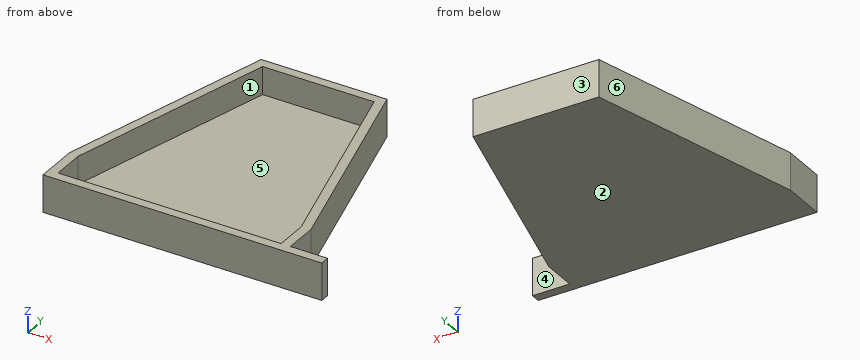
from build123d import *

# Parameters (mm, degrees)
F2_DEPTH = 3.175
F3_DEPTH = 12.7
F4_W     = 3.175
F4_H     = 12.7
F5_DEPTH = 12.7


with BuildPart() as f2:
    # F0 (on Top) → F2 (new body)
    with BuildSketch(Plane.XY):
        Polygon((-38.1, -30.1625), (-38.1, -41.275), (38.1, -41.275), (38.1, -30.1625), (19.05, 41.275), (-19.05, 41.275), align=None)
    extrude(amount=F2_DEPTH)

    # F1 (on face) → F3 (join)
    with BuildSketch(Plane.XY):
        Polygon((21.489284, 44.45), (-21.489284, 44.45), (-41.275, -29.746436), (-41.275, -44.45), (41.275, -44.45), (41.275, -29.746436), align=None)
        Polygon((-38.1, -41.275), (-38.1, -30.1625), (-19.05, 41.275), (19.05, 41.275), (38.1, -30.1625), (38.1, -41.275), align=None, mode=Mode.SUBTRACT)
    extrude(amount=F3_DEPTH)

    # F4 (on face) → F5 (join)
    with BuildSketch(Plane.YZ.offset(41.275)):
        with Locations((-42.8625, 6.35)):
            Rectangle(F4_W, F4_H)
    extrude(amount=F5_DEPTH)


solid = f2.part
Read the model definition and answer for the solid it produces. Units are mm, in the model's axes. Face numbers are marked on the shaded views. A direction names the side the tool comes from. Give positions to 0.01 mm unless a question says otherwise; leave off trailing zeros. Write each loop counter-clockwise with the first axis right and the second up, starting at its lowest first coordinate (ties: lowest second). Pieces come first, ordered by that corner, then holes. Notation, with made-up numbers: M 46,47 L 75,47 A20 cw 75,80 Z; hole C 39,18 d6. An arc over 180 degrees is marked long. One line per item, written item: value. Start each with the question number.
(1) Find section B-B (x = -7). Determine the outline of the cut face in (y, z) (3 decimals).
(2) A tool of negligible diameter and unlimited length cuts with its end or side. For the marked faces 4, 5 and 6, from which of +Z, -Z, +X, -X, +Y, -Y can it reach the whole face along a straight path? Write none if from no direction.
(3) Flat-ended cylindrical pins translate along their axes: pin 1 Ø6 at (y, z) = (-37, 8.5) entering from +X (3 decimals); pin 2 Ø4 at (y, z) = (25, 10.5) entering from -X; pin 3 Ø4 at (y, z) = (-2, 5) entering from +X. Find the tip coordinate at first contact, or state that the pin passes through.
(4) Find section C-C (y = -38). Determine the outline of the cut face in (x, z) (3 decimals), plus the area to 3 significant figures.
(5) Determine the mould class of the marked faces 1, 2 and 3 for opening direction Y: pulls with the +Y half, pulls with the -Y half, needs draft (parallel to the pull), parting line crosses it, or undercut.
(6) Find the intervals of material crossed by line 1 (Y direction, x = 10.5, z = 4.5) (3 decimals); line 2 (X direction, y = -25, z = 12.25); line 3 (X direction, y = -2.5, z = 8.5), in increasing order.
Results below:
1. outline: M -44.45,0 L 44.45,0 L 44.45,12.7 L 41.275,12.7 L 41.275,3.175 L -41.275,3.175 L -41.275,12.7 L -44.45,12.7 Z
2. face 4: +Z, -Z, +X, +Y
2. face 5: +Z
2. face 6: +Z, -Z, -X, +Y
3. pin 1: stops at x = 41.275
3. pin 2: stops at x = -27.21
3. pin 3: stops at x = 34.41
4. outline: M -41.275,0 L 41.275,0 L 41.275,12.7 L 38.1,12.7 L 38.1,3.175 L -38.1,3.175 L -38.1,12.7 L -41.275,12.7 Z
4. area: 323 mm^2
5. face 1: undercut
5. face 2: needs draft
5. face 3: pulls with the +Y half
6. line 1: y = -44.45 to -41.275, 41.275 to 44.45
6. line 2: x = -40.01 to -36.72, 36.72 to 40.01
6. line 3: x = -34.01 to -30.72, 30.72 to 34.01
